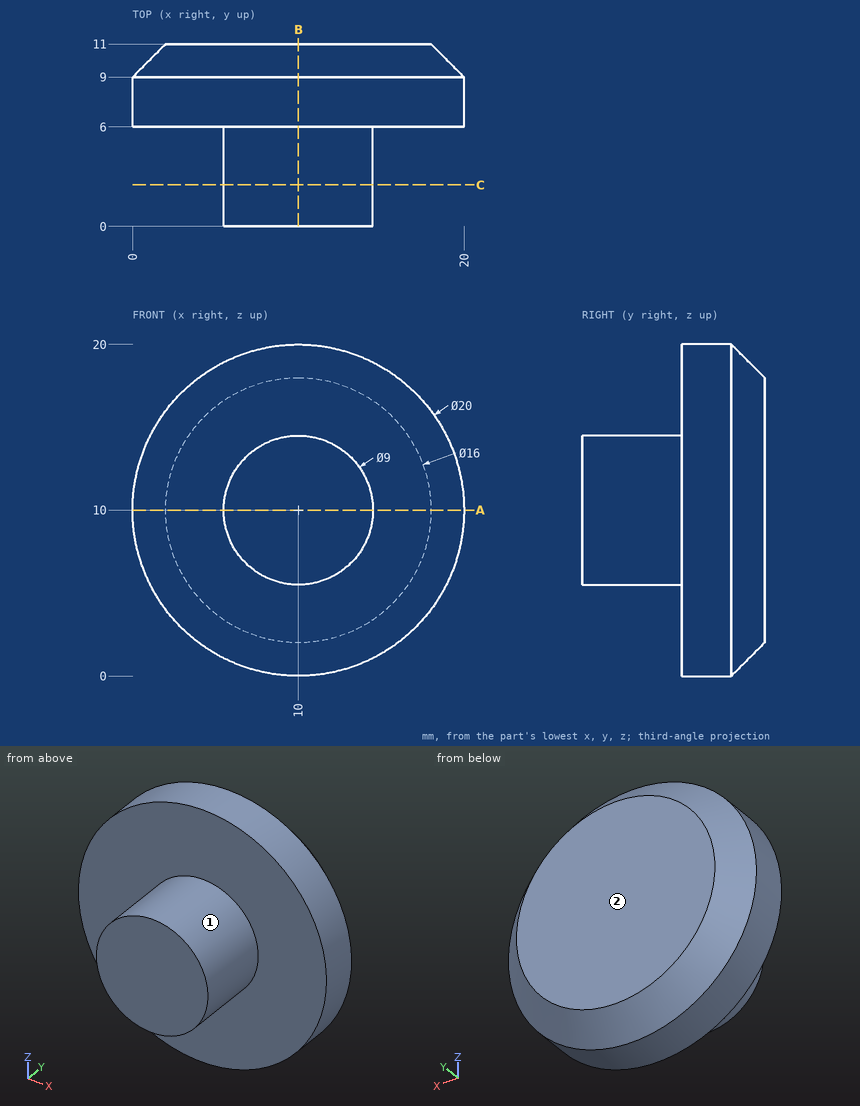
Source: three-view drawing plus pictorial views. Frame: mm from the lowest corner of the part. A direction names the side the tool comes from. Give positions to 0.01 mm unless a question says otherwise; leave off trailing zeros. Write each loop counter-clockwise with the first axis right and the second up, starting at its lowest first coordinate (ties: lowest second). Pieces come first, ordered by that corner, then holes.
(1) Cut plane A-A, the plane z = 10. Return loops of the section in (x, y), then the cut area to 3 significant figures.
(2) Cut plane C-C, the plane y = 2.5. Return loops of the section in (x, z), then the cut area to 3 significant figures.
(3) Ray query, line 1 (Y direction, x = 2.5, z = 11.75); line 2 (Z direction, x = 10.25, y = 8); line 3 (X direction, y = 1.25, z = 7.75). Return the intervals inside material, ascending.
(4) Cut plane B-B, the plane x = 10. Return loops of the section in (y, z), then the cut area to 3 significant figures.
(5) First-contact query: P1, Ø2, axis at x = 2.5, z = 6, coming from the -Y side; P2, Ø6, axis at x = 8.5, y = 1.5, coming from the -Z side; P3, Ø1, axis at x = 2.5, y = 6, coming from the +Z side; P4, Ø5, axis at x = 15.5, z = 7, coming from the -Y side. Flat tips, straight axial feed; report the tip coordinate or a pass-through.
(6) Access query for the marked faces 1 and 2. Directions: +Z, -Z, +X, -X, +Y, -Y. A direction counts if a zero-diameter tool reaches every point of the face in a straight line with its end or side. Return the directions, or none.
Values follow:
1. outline: (0, 6) - (5.5, 6) - (5.5, 0) - (14.5, 0) - (14.5, 6) - (20, 6) - (20, 9) - (18, 11) - (2, 11) - (0, 9) - close
1. area: 150 mm2
2. outline: circle Ø9 at (10, 10)
2. area: 63.6 mm2
3. line 1: y = 6 to 11
3. line 2: z = 0 to 20
3. line 3: x = 6.1 to 13.9
4. outline: (0, 5.5) - (6, 5.5) - (6, 0) - (9, 0) - (11, 2) - (11, 18) - (9, 20) - (6, 20) - (6, 14.5) - (0, 14.5) - close
4. area: 150 mm2
5. P1: stops at y = 6
5. P2: stops at z = 5.5
5. P3: stops at z = 17.14
5. P4: stops at y = 0
6. face 1: -Y
6. face 2: +Z, -Z, +X, -X, +Y
